The drawing under review shows one solid part. Ordinate dimensions are in mm from its lowest x, y, z. A direction names the side the tool comes from. Coordinates: 2 decimals unless noted, no trailing zeros. Order: outer loops, then holes, each group sorted by start corner. A loop starts at its lowest first (then second) coordinate and runs counter-clockwise, first axis right, second up.
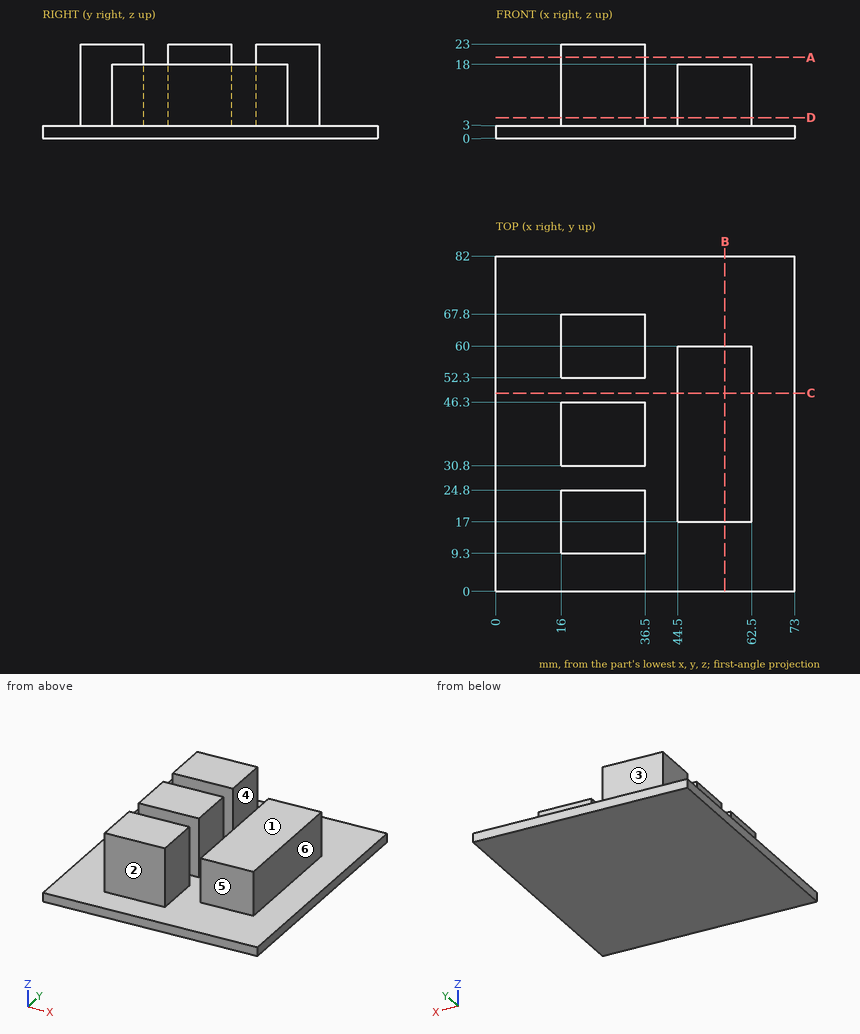
1. Add section B-B (x = 56). Give the boundary of the cut face in (y, z).
2. Mouldability with a two-part tool opening along X and no side actions: class the marked faces 4, 5 and 6 as pulls with the +X half, pulls with the -X half, needs draft (parallel to the pull), parting line crosses it, or undercut.
3. To check wall thickness, follow line 1 (Y direction, x = 32, z = 19); line 2 (X direction, y = 33, z = 11.25); line 3 (Z direction, x = 40, y = 19). State the ranges of each line that lie inside material, in increasing order.
4. For the marked faces 1, 2 and 3, list the 3-axis set-ups (+Z, -Z, +X, -X, +Y, -Y) from which the entire face can be reached by the end or side of a thin tool; tool diameter is ignored.
5. Insertion check: pin 1 (7.5 mm diameter, centred on y = 38.5, z = 9.5, fed in from -X); pin 2 (10 mm diameter, centred on x = 55, z = 14.5, fed in from -Y); pin 3 (6 mm diameter, centred on x = 7.5, y = 24, fed in from +Z). Each pin has a flat end and moves straight along its axis. Give the tip position at first contact, or say it passes through.
6. Add section C-C (y = 48.5). Give the boundary of the cut face in (x, z), and give its area (3 significant figures).
7. Add section D-D (z = 5). Give the boundary of the cut face in (x, y), and give its area (3 significant figures).
8. Add section A-A (z = 19.75). Give the boundary of the cut face in (x, y), and give its area (3 significant figures).
Solution:
1. outline: (0, 0) - (82, 0) - (82, 3) - (60, 3) - (60, 18) - (17, 18) - (17, 3) - (0, 3) - close
2. face 4: undercut
2. face 5: needs draft
2. face 6: pulls with the +X half
3. line 1: y = 9.3 to 24.8, 30.8 to 46.3, 52.3 to 67.8
3. line 2: x = 16 to 36.5, 44.5 to 62.5
3. line 3: z = 0 to 3
4. face 1: +Z, +X, +Y, -Y
4. face 2: +Z, +X, -X, -Y
4. face 3: +Z, +X, -X, +Y
5. pin 1: stops at x = 16
5. pin 2: stops at y = 17
5. pin 3: stops at z = 3
6. outline: (0, 0) - (73, 0) - (73, 3) - (62.5, 3) - (62.5, 18) - (44.5, 18) - (44.5, 3) - (0, 3) - close
6. area: 489 mm2
7. outline: (16, 9.3) - (36.5, 9.3) - (36.5, 24.8) - (16, 24.8) - close; (16, 30.8) - (36.5, 30.8) - (36.5, 46.3) - (16, 46.3) - close; (16, 52.3) - (36.5, 52.3) - (36.5, 67.8) - (16, 67.8) - close; (44.5, 17) - (62.5, 17) - (62.5, 60) - (44.5, 60) - close
7. area: 1,730 mm2
8. outline: (16, 9.3) - (36.5, 9.3) - (36.5, 24.8) - (16, 24.8) - close; (16, 30.8) - (36.5, 30.8) - (36.5, 46.3) - (16, 46.3) - close; (16, 52.3) - (36.5, 52.3) - (36.5, 67.8) - (16, 67.8) - close
8. area: 953 mm2
